Source: CAD feature listing. Evaluate the final solid. Frame: model axes, mm. Face numbers are marked on the shaded views. A direction names the side the tool comes from. Round coordinates to 2 decimals unless told otherwise and drop trailing zeros. Loops run counter-clockwise (first coordinate to the right, second up) from the corner with the lowest first, then second, coordinate; pieces in that order, holes last. Notation, with made-up numbers: (-29.5, 85) -> (-6.5, 85) arc R21 ccw to (-6.5, 110) -> close; hole circle Ø7 at (1.5, 12.25). An arc over 180 degrees is marked (long way). Return JSON: item names as keys, results as strings. Group by question number.
```python
from build123d import *

# Parameters (mm, degrees)
F0_W      = 60
F0_H      = 30
F1_DEPTH  = 10
F2_W      = 10
F2_H      = 30
F3_DEPTH  = 37.5
F5_DEPTH  = 60.001
F6_R      = 7.5
F7_DEPTH  = 60.001
F9_DEPTH  = 2.5
F11_DEPTH = 10
F12_R     = 10
F13_DEPTH = 25


with BuildPart() as f1:
    # F0 (on Top) → F1 (new body)
    with BuildSketch(Plane.XY):
        Rectangle(F0_W, F0_H)
    extrude(amount=F1_DEPTH)

    # F2 (on face) → F3 (join)
    with BuildSketch(Plane.XY.offset(10)):
        with Locations((-25, 0)):
            Rectangle(F2_W, F2_H)
        with Locations((25, 0)):
            Rectangle(F2_W, F2_H)
    extrude(amount=F3_DEPTH)

    # F4 (on face) → F5 (cut, through all)
    with BuildSketch(Plane(origin=(-30, 0, 0), x_dir=(0, -1, 0), z_dir=(-1, 0, 0))):
        with BuildLine():
            ThreePointArc((-15, 32.5), (-10.6066017178, 43.1066017178), (0, 47.5))
            Line((0, 47.5), (-15, 47.5))
            Line((-15, 47.5), (-15, 32.5))
        make_face()
        with BuildLine():
            ThreePointArc((0, 47.5), (10.6066017178, 43.1066017178), (15, 32.5))
            Line((15, 32.5), (15, 47.5))
            Line((15, 47.5), (0, 47.5))
        make_face()
    extrude(amount=-F5_DEPTH, mode=Mode.SUBTRACT)

    # F6 (on face) → F7 (cut, through all)
    with BuildSketch(Plane(origin=(-30, 0, 0), x_dir=(0, -1, 0), z_dir=(-1, 0, 0))):
        with Locations((0, 32.5)):
            Circle(F6_R)
    extrude(amount=-F7_DEPTH, mode=Mode.SUBTRACT)

    # F8 (on face) → F9 (join)
    with BuildSketch(Plane(origin=(0, 0, 0), x_dir=(1, 0, 0), z_dir=(0, 0, -1))):
        with BuildLine():
            Line((-8, 15), (8, 15))
            ThreePointArc((8, 15), (0, 17), (-8, 15))
        make_face()
        with BuildLine():
            ThreePointArc((8, -15), (14.5773797371, -8.7464278423), (17, 0))
            ThreePointArc((17, 0), (14.5773797371, 8.7464278423), (8, 15))
            Line((8, 15), (-8, 15))
            ThreePointArc((-8, 15), (-17, 0), (-8, -15))
            Line((-8, -15), (8, -15))
        make_face()
        with BuildLine():
            ThreePointArc((-8, -15), (0, -17), (8, -15))
            Line((8, -15), (-8, -15))
        make_face()
    extrude(amount=F9_DEPTH)

    # F10 (on face) → F11 (join)
    with BuildSketch(Plane.XY.offset(10)):
        with BuildLine():
            Line((-13.2287565553, 15), (13.2287565553, 15))
            ThreePointArc((13.2287565553, 15), (0, 20), (-13.2287565553, 15))
        make_face()
        with BuildLine():
            Line((13.2287565553, -15), (-13.2287565553, -15))
            ThreePointArc((-13.2287565553, -15), (0, -20), (13.2287565553, -15))
        make_face()
    extrude(amount=-F11_DEPTH)

    # F12 (on face) → F13 (cut)
    with BuildSketch(Plane.XY.offset(10)):
        Circle(F12_R)
    extrude(amount=-F13_DEPTH, mode=Mode.SUBTRACT)


solid = f1.part
```
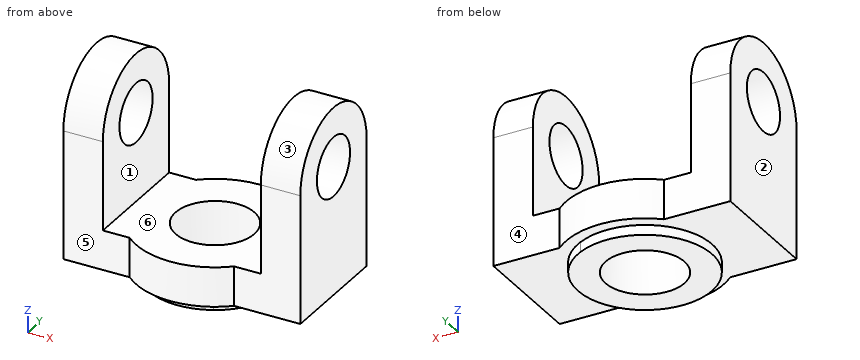
(1) Set-up query: the marked faces 4, 5 and 6. Return all of +Z, -Z, +X, -X, +Y, -Y with unobstructed straight access to the full face (end or side cutting, diameter ignored); none if empty.
(2) Cut plane B-B (y = 4). Return loops of the section in (x, z), and give its area (3 significant figures).
(3) Cut plane D-D (x = -23.5). Return loops of the section in (y, z).
(4) Ray query, line 1 (X direction, y = -14, z = 12); line 2 (Z direction, x = 25, y = 0); line 3 (Z direction, x = -8, y = 10). Return the intervals inside material, ascending.
(5) Mould query, pull axis X, two halves, no side actions, for the marked faces 1, 2 and 3. Classes: released by +X, released by -X, zero draft, split by the parting line, or undercut.
(6) Pin query (flat end, axial travel): pin 1 (1.5 mm diameter, centred on x = 22.5, y = -2.5, fed in from -Z); pin 2 (5 mm diameter, centred on x = -19, z = 20.5, fed in from +Y); pin 3 (12 mm diameter, centred on x = -2.5, y = 6.5, fed in from +Z). Return the tip coordinate at first contact, or that it passes through.
(7) Cut plane C-C (z = 22.5). Return loops of the section in (x, y).
(8) Cut plane A-A (x = 0). Return loops of the section in (y, z).
Answers follow:
{
 "1": {"face 4": "+Z, -Z, +X, +Y", "face 5": "+Z, -Z, -X, -Y", "face 6": "+Z, +Y, -Y"},
 "2": {"outline": "(-30, 0) -> (-16.52, 0) -> (-16.52, -2.5) -> (-9.17, -2.5) -> (-9.17, 10) -> (-20, 10) -> (-20, 26.16) -> (-30, 26.16) -> close; (-30, 38.84) -> (-20, 38.84) -> (-20, 46.96) -> (-30, 46.96) -> close; (9.17, -2.5) -> (16.52, -2.5) -> (16.52, 0) -> (30, 0) -> (30, 26.16) -> (20, 26.16) -> (20, 10) -> (9.17, 10) -> close; (20, 38.84) -> (30, 38.84) -> (30, 46.96) -> (20, 46.96) -> close", "area": "939 mm^2"},
 "3": {"outline": "(-15, 0) -> (15, 0) -> (15, 32.5) arc R15 ccw to (-15, 32.5) -> close; hole circle Ø15 at (0, 32.5)"},
 "4": {"line 1": "-30 to -20, 20 to 30", "line 2": "0 to 25, 40 to 47.5", "line 3": "-2.5 to 10"},
 "5": {"face 1": "undercut", "face 2": "released by -X", "face 3": "zero draft"},
 "6": {"pin 1": "z = 0", "pin 2": "y = 15", "pin 3": "z = 10"},
 "7": {"outline": "(-30, -15) -> (-20, -15) -> (-20, 15) -> (-30, 15) -> close; (20, -15) -> (30, -15) -> (30, 15) -> (20, 15) -> close"},
 "8": {"outline": "(-20, 0) -> (-17, 0) -> (-17, -2.5) -> (-10, -2.5) -> (-10, 10) -> (-20, 10) -> close; (10, -2.5) -> (17, -2.5) -> (17, 0) -> (20, 0) -> (20, 10) -> (10, 10) -> close"}
}
